Read the model definition and answer for the solid it produces. Units are mm, in the model's axes. A direction names the side the tool comes from. Round coordinates to 2 decimals unless told otherwise and drop trailing zeros. Order: outer loops, then holes, each group sorted by start corner. A loop starts at its lowest first (then second) coordinate and runs counter-clockwise, first axis right, second up. Notation, with made-up numbers: (35.25, 84) -> (65.25, 84) arc R22 cw to (65.25, 116) -> close; hole circle Ø7 at (18.25, 17.5). An arc over 180 degrees is marked (long way). Answer as a JSON object with one key per item and string values. Group by question number.
Item 1: Section C-C, the plane x = -82 is taken. Write down the section's boundary in (y, z).
Item 2: Section A-A, the plane y = 0 is taken. Write down the section's boundary in (x, z) (3 decimals).
Item 3: Consider probe 1 along Z at (x, y) = (-134, 0) (3 decimals); probe 2 along Y at (x, z) = (56.5, 0.5); probe 3 along X at (y, z) = (-3.25, 5.5). Determine where each line is inside the solid, lowest interval first. Write a range as from..to.
Item 4: Given P1, Ø2, axis at y = 0, z = -1, coming from the -X side; P2, Ø1.5, axis at x = 76.5, z = -2, coming from the +Y side; P3, Ø10, axis at x = 83.5, y = -9, coming from the +Z side, each flat-ended and moving along its own axis, determine where each tip first touches the part or whether it passes through.
Item 5: The mould has two halves that part along Y. Classify faces 1 (the flat face through (140.97, 0, 0)), 2 (the cylindrical face through (137.589, -7.559, -5.796)), 3 (the cylindrical face through (-135.961, 7.559, -5.796)): pulls with the +Y half, pulls with the -Y half, needs draft (parallel to the pull), parting line crosses it, or undercut.
Item 6: For faces 4 (the cylindrical face through (-1.51, -8.87, -6.8)), 5 (the flat face through (134.112, 9.2, -3)), 6 (the flat face through (-130.81, 0, 0)), determine the directions among +Z, -Z, +X, -X, +Y, -Y from which every point of the face is accessible in a straight line to the end or side of a thin tool.
from build123d import *

# Parameters (mm, degrees)
F0_R     = 11.176
F1_DEPTH = 140.97
F2_R     = 11.176
F2_R_2   = 9.525
F3_DEPTH = 6.858
F4_SIZE  = 0.762
F5_R     = 9.525
F6_DEPTH = 10.16


with BuildPart() as f1:
    # F0 (on Right) → F1 (new body, symmetric)
    with BuildSketch(Plane.YZ):
        Circle(F0_R)
    extrude(amount=F1_DEPTH, both=True)

    # F2 (on face) → F3 (cut)
    with BuildSketch(Plane.YZ.offset(140.97)):
        Circle(F2_R)
        Circle(F2_R_2, mode=Mode.SUBTRACT)
    extrude(amount=-F3_DEPTH, mode=Mode.SUBTRACT)

    # F4
    f4_edges = [f1.edges().sort_by_distance(p)[0] for p in [
        (-140.97, -11.176, 0),
        (134.112, -11.176, 0),
    ]]
    chamfer(f4_edges, length=F4_SIZE)

    # F5 (on face) → F6 (cut)
    with BuildSketch(Plane(origin=(-140.97, 0, 0), x_dir=(0, -1, 0), z_dir=(-1, 0, 0))):
        Circle(F5_R)
    extrude(amount=-F6_DEPTH, mode=Mode.SUBTRACT)


solid = f1.part
Values found:
{
 "1": {"outline": "circle Ø22.35 at (0, 0)"},
 "2": {"outline": "(-140.97, -10.414) -> (-140.208, -11.176) -> (133.35, -11.176) -> (134.112, -10.414) -> (134.112, -9.525) -> (140.97, -9.525) -> (140.97, 9.525) -> (134.112, 9.525) -> (134.112, 10.414) -> (133.35, 11.176) -> (-140.208, 11.176) -> (-140.97, 10.414) -> (-140.97, 9.525) -> (-130.81, 9.525) -> (-130.81, -9.525) -> (-140.97, -9.525) -> close"},
 "3": {"probe 1": "-11.176..-9.525, 9.525..11.176", "probe 2": "-11.16..11.16", "probe 3": "-130.81..140.97"},
 "4": {"P1": "x = -130.81", "P2": "y = 11.11", "P3": "z = 10.44"},
 "5": {"face 1": "needs draft", "face 2": "parting line crosses it", "face 3": "undercut"},
 "6": {"face 4": "+X, -X", "face 5": "+X", "face 6": "-X"}
}
